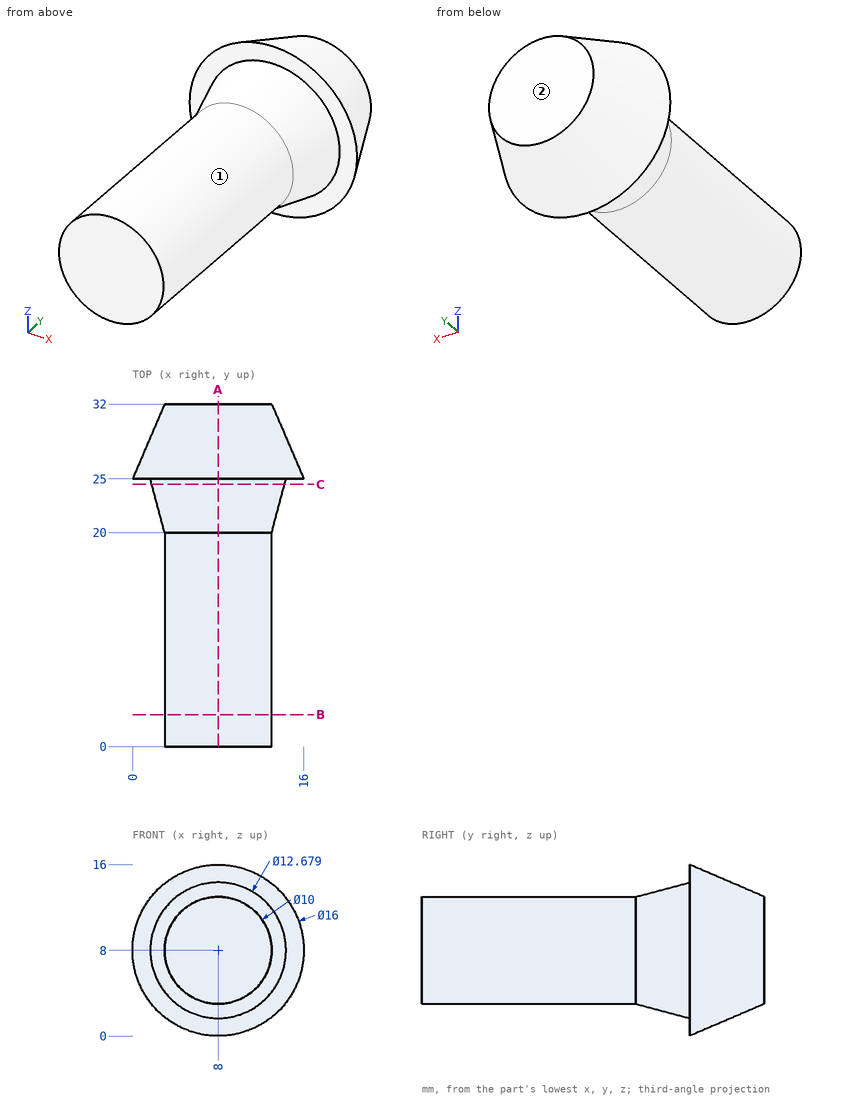
Input: dimensioned drawing with shaded views. Units: mm. Origin: part minimum x, y, z. A direction names the side the tool comes from. Give positions to 0.01 mm unless a question says otherwise; leave off trailing zeros. Order: outer loops, then holes, each group sorted by start corner. A loop starts at its lowest first (then second) coordinate and runs counter-clockwise, first axis right, second up. Notation, with made-up numbers: (61, 4.5) -> (92, 4.5) arc R37 ccw to (92, 43.5) -> close; hole circle Ø5 at (-20.5, 28). An arc over 180 degrees is marked (long way). Write item = value, one per line.
Item 1: Section query C-C (y = 24.5). Output: boundary loops of the cut face in (x, z) (1 decimal), then the cut area to 3 significant figures.
Check result:
outline = circle Ø12.4 at (8, 8)
area = 121 mm²
Item 2: Section query B-B (y = 3). Output: boundary loops of the cut face in (x, z).
Check result:
outline = circle Ø10 at (8, 8)
Item 3: Contact query for flat-ended pins moving along their axis: pin 1 (1.5 mm diameter, centred on x = 6, z = 13.5, fed in from +Y) (1 decimal); pin 2 (4 mm diameter, centred on y = 20.5, z = 6.5, fed in from +X); pin 3 (1.5 mm diameter, centred on x = 9.5, y = 22, fed in from +Z). Output: stop coordinate, or through.
Check result:
pin_1 = 31.8
pin_2 = 13.58
pin_3 = 13.6
Item 4: Ray query, probe 1 along Z at (x, y) = (8, 6); probe 2 along X at (y, z) = (13.5, 10.75) (1 decimal); probe 3 along Z at (x, y) = (13, 24) (1 decimal). Return the intervals inside material, ascending.
Check result:
probe_1 = 3 to 13
probe_2 = 3.8 to 12.2
probe_3 = 4.6 to 11.4
Item 5: Section query A-A (x = 8). Output: boundary loops of the cut face in (y, z), then the cut area to 3 significant figures.
Check result:
outline = (0, 3) -> (20, 3) -> (25, 1.66) -> (25, 0) -> (32, 3) -> (32, 13) -> (25, 16) -> (25, 14.34) -> (20, 13) -> (0, 13) -> close
area = 348 mm²
Item 6: Set-up query: the marked faces 1 and 2. Return all of +Z, -Z, +X, -X, +Y, -Y with unobstructed straight access to the full face (end or side cutting, diameter ignored); none if empty.
Check result:
face_1 = -Y
face_2 = +Z, -Z, +X, -X, +Y
